Autodesk Inventor part; units mm, degrees
ref_plane "YZ Plane" through (0, 0, 0) normal (1, 0, 0) x (0, 1, 0)
ref_plane "XZ Plane" through (0, 0, 0) normal (0, 1, 0) x (-1, 0, 0)
ref_plane "XY Plane" through (0, 0, 0) normal (0, 0, 1) x (1, 0, 0)
sketch "Sketch1" plane through (0, 0, 0) normal (0, 1, 0) x (-1, 0, 0)
  line L0 (101.6, 38.1) -> (-101.6, 38.1) construction
  line L1 (-101.6, 38.1) -> (-101.6, -38.1) construction
  line L2 (-101.6, -38.1) -> (101.6, -38.1) construction
  line L3 (101.6, -38.1) -> (101.6, 38.1) construction
  line L4 (101.6, 38.1) -> (-101.6, -38.1) construction
  line L5 (-101.6, 38.1) -> (101.6, -38.1) construction
  line L6 (-28.575, 66.675) -> (28.575, 66.675) construction
  line L7 (28.575, 66.675) -> (28.575, 9.525)
  line L8 (28.575, 9.525) -> (-28.575, 9.525) construction
  line L9 (-28.575, 9.525) -> (-28.575, 66.675)
  line L10 (-28.575, 66.675) -> (28.575, 9.525) construction
  line L11 (28.575, 66.675) -> (-28.575, 9.525) construction
  circle A0 centre (-38.1, 50.8) radius 3.175
  line L12 (0, 38.1) -> (0, -38.1) construction
  circle A1 centre (-38.1, 50.8) radius 9.525
  line L13 (-38.1, 60.325) -> (-28.575, 60.325)
  circle A2 centre (38.1, 50.8) radius 3.175
  circle A3 centre (38.1, 50.8) radius 9.525
  line L14 (38.1, 60.325) -> (28.575, 60.325)
  circle A4 centre (-76.2, -38.1) radius 1.7526
  circle A5 centre (-95.25, 3.175) radius 1.7526
  circle A6 centre (76.2, -38.1) radius 1.7526
  circle A7 centre (95.25, 3.175) radius 1.7526
  line L15 (-101.6, -38.1) -> (-101.6, 6.35)
  line L16 (-101.6, 6.35) -> (-44.4797, 57.8728)
  line L17 (101.6, -38.1) -> (101.6, 6.35)
  line L18 (101.6, 6.35) -> (44.4797, 57.8728)
  line L19 (-42.6417, 42.4275) -> (-87.975, 1.5367) construction
  line L20 (-87.975, 1.5367) -> (-87.975, -38.1)
  line L21 (87.975, -38.1) -> (87.975, 1.5367)
  line L22 (87.975, 1.5367) -> (42.6417, 42.4275) construction
  line L23 (0, -38.1) -> (-95.25, -38.1) construction
  line L24 (0, -38.1) -> (95.25, -38.1) construction
  circle A8 centre (-60.325, 35.0287) radius 1.7526
  circle A9 centre (-33.3375, 31.75) radius 1.7526
  line L25 (-38.1, 0) -> (-38.1, 41.275)
  line L26 (-38.1, 0) -> (0, 0) construction
  circle A10 centre (60.325, 35.0287) radius 1.7526
  circle A11 centre (33.3375, 31.75) radius 1.7526
  line L27 (38.1, 0) -> (38.1, 41.275)
  line L28 (38.1, 0) -> (0, 0) construction
  line L29 (-87.975, 0) -> (-65.115, 0)
  line L30 (-65.115, 0) -> (-65.115, -31.75)
  line L31 (-65.115, -31.75) -> (-87.975, -31.75)
  line L32 (-101.6, -38.1) -> (101.6, -38.1) construction
  line L33 (101.6, -38.1) -> (101.6, 19.05)
  line L34 (101.6, 19.05) -> (-101.6, 19.05) construction
  line L35 (-101.6, 19.05) -> (-101.6, -38.1)
  line L36 (-101.6, 19.05) -> (-87.5203, 19.05) construction
  line L37 (87.5203, 19.05) -> (101.6, 19.05) construction
  circle A12 centre (-38.1, 0) radius 3.175 construction
  circle A13 centre (-38.1, 0) radius 6.35 construction
  circle A14 centre (38.1, 0) radius 3.175 construction
  circle A15 centre (38.1, 0) radius 6.35 construction
  circle A16 centre (28.575, 9.525) radius 1.7526
  circle A17 centre (28.575, 9.525) radius 4.7625
  arc A18 (17.0773, 9.525) -> (28.575, 21.0227) centre (17.0773, 21.0227) ccw
  circle A19 centre (-28.575, 9.525) radius 1.7526
  circle A20 centre (-28.575, 9.525) radius 4.7625
  arc A21 (-28.575, 21.0227) -> (-17.0773, 9.525) centre (-17.0773, 21.0227) ccw
  arc A22 (31.4325, 5.715) -> (38.1, 19.05) centre (21.4312, 19.05) ccw
  arc A23 (-38.1, 19.05) -> (-31.4325, 5.715) centre (-21.4312, 19.05) ccw
  line L38 (-61.94, -38.1) -> (-61.94, 25.0204)
  line L39 (87.975, 0) -> (65.115, 0)
  line L40 (65.115, 0) -> (65.115, -31.75)
  line L41 (65.115, -31.75) -> (87.975, -31.75)
  line L42 (61.94, -38.1) -> (61.94, 25.0204)
  line L43 (-28.575, 4.7625) -> (28.575, 4.7625)
  line L44 (101.6, -31.75) -> (-101.6, -31.75)
  line L45 (-101.6, -31.75) -> (-101.6, -44.45) construction
  line L46 (-101.6, -44.45) -> (101.6, -44.45)
  line L47 (101.6, -44.45) -> (101.6, -31.75) construction
  circle A24 centre (0, -38.1) radius 1.7526
  circle A25 centre (38.1, -38.1) radius 1.7526
  circle A26 centre (-38.1, -38.1) radius 1.7526
  line L48 (101.6, -38.1) -> (76.2, -44.45)
  line L49 (-101.6, -38.1) -> (-76.2, -44.45)
  line L50 (76.2, -38.1) -> (76.2, -44.45) construction
  line L51 (-76.2, -38.1) -> (-76.2, -44.45) construction
  line L52 (59.1924, 41.2769) -> (32.488, 36.4361)
  circle A27 centre (60.325, 35.0287) radius 6.35
  circle A28 centre (33.3375, 31.75) radius 4.7625
  line L53 (-59.1924, 41.2769) -> (-32.488, 36.4361)
  circle A29 centre (-60.325, 35.0287) radius 6.35
  circle A30 centre (-33.3375, 31.75) radius 4.7625
  line L54 (-87.975, 0) -> (-65.115, 0)
  line L55 (-65.115, 0) -> (-65.115, -3.175)
  line L56 (-65.115, -3.175) -> (-87.975, -3.175)
  line L57 (-87.975, -3.175) -> (-87.975, 0)
  line L58 (-65.115, -15.875) -> (-87.975, -15.875) construction
  line L59 (-65.115, -28.575) -> (-87.975, -28.575)
  line L60 (-84.8, -38.1) -> (-84.8, 0.1248)
  line L61 (65.115, -3.175) -> (87.975, -3.175)
  line L62 (65.115, -15.875) -> (87.975, -15.875) construction
  line L63 (65.115, -28.575) -> (87.975, -28.575)
  line L64 (84.8, -38.1) -> (84.8, 0.1248)
  line L65 (-31.75, -31.75) -> (31.75, -31.75)
  line L66 (31.75, -31.75) -> (31.75, 0)
  line L67 (31.75, 0) -> (-31.75, 0)
  line L68 (-31.75, 0) -> (-31.75, -31.75)
  circle A31 centre (71.465, 12.7) radius 3.175
  circle A32 centre (-71.465, 12.7) radius 3.175
  line L69 (-17.0773, 9.525) -> (17.0773, 9.525)
  point P0 (28.575, 38.1)
  point P1 (-28.575, 38.1)
  point P2 (28.575, 60.325)
  point P3 (44.4797, 57.8728)
  point P4 (101.6, -15.875)
  point P5 (38.1, 41.275)
  point P6 (-87.975, -31.75)
  point P7 (-101.6, 6.35)
  point P8 (101.6, 6.35)
  point P9 (31.75, 0)
  point P10 (38.1, 6.35)
  point P11 (-38.1, 6.35)
  point P12 (-31.75, 0)
  point P13 (87.975, 0)
  point P14 (61.94, 25.0204)
  point P15 (-17.0773, 9.525)
  point P16 (-28.575, 21.0227)
  point P17 (-38.1, 19.05)
  point P18 (-31.4325, 5.715)
  point P19 (-21.8502, 0)
  point P20 (21.8502, 0)
  point P21 (-25.2074, 12.8926)
  point P22 (-28.575, 14.2875)
  point P23 (-23.8125, 9.525)
  point P24 (-28.575, 50.8)
  point P25 (25.2074, 12.8926)
  point P26 (28.575, 14.2875)
  point P27 (23.8125, 9.525)
  point P28 (28.575, 50.8)
  point P29 (26.8224, 9.525)
  point P30 (28.575, 11.2776)
  point P31 (61.94, -31.75)
  point P32 (-61.94, -31.75)
  point P33 (-28.575, 31.75)
  point P34 (-64.5781, 39.7439)
  point P35 (64.5781, 39.7439)
  point P36 (28.575, 31.75)
  point P37 (-84.8, -3.175)
  point P38 (-84.8, -28.575)
  point P39 (84.8, -3.175)
  point P40 (84.8, -28.575)
  point P41 (31.75, -31.75)
  point P42 (-101.6, -31.75)
  point P43 (31.75, -31.75)
  point P44 (-26.8224, 9.525)
  point P45 (-28.575, 11.2776)
  point P46 (-39.8526, -38.1)
  point P47 (-36.3474, -38.1)
  point P48 (-1.7526, -38.1)
  point P49 (1.7526, -38.1)
  point P50 (36.3474, -38.1)
  point P51 (39.8526, -38.1)
  dimension "d0" = 203.2
  dimension "d1" = 76.2
  dimension "d4" = 57.15
  dimension "d6" = 6.35
  dimension "d7" = 38.1
  dimension "d8" = 19.05
  dimension "d10" = 3.5052
  dimension "d11" = 3.5052
  dimension "d12" = 0
  dimension "d14" = 25.4
  dimension "d15" = 6.35
  dimension "d20" = 50.8
  dimension "d21" = 41.275
  dimension "d22" = 44.45
  dimension "d24" = 12.7
  dimension "d25" = 13.625
  dimension "d26" = 12.7
  dimension "d27" = 13.625
  dimension "d31" = 3.5052
  dimension "d32" = 3.5052
  dimension "d33" = 6.35
  dimension "d34" = 31.75
  dimension "d35" = 4.7625
  dimension "d36" = 22.225
  dimension "d37" = 9.525
  dimension "d39" = 31.75
  dimension "d40" = 6.35
  dimension "d42" = 57.15
  dimension "d43" = 6.35
  dimension "d44" = 9.525
  dimension "d45" = 9.525
  dimension "d46" = 12.7
  dimension "d104" = 3.5052
  dimension "d105" = 9.525
  dimension "d106" = 3.175
  dimension "d107" = 22.86
  dimension "d123" = 88.9
  dimension "d124" = 12.7
  dimension "d125" = 3.5052
  dimension "d126" = 3.5052
  dimension "d127" = 38.1
  dimension "d128" = 28.575
  dimension "d129" = 3.175
  dimension "d130" = 3.175
  dimension "d131" = 31.75
  dimension "d132" = 31.75
  dimension "d133" = 31.75
  dimension "d135" = 6.35
  dimension "d136" = 12.7
  dimension "d137" = 9.525
extrude "Extrusion1" add sketch "Sketch1" along normal blind 3.175 contours A28 L27 A22 A17 L7 | A28 | L7 A17 A18 | L52 L27 A28 | L27 L52 A27 L18 L17 L44 L21 L39 L40 L66 L67 L68 L30 L29 L20 L15 L16 A29 L53 L25 A23 A20 L43 A17 A22 | A27 | A17 | A17 L43 A20 A21 L69 A18 | L17 L48 L46 L49 L15 L44 L31 L41 | A20 | L41 L64 L63 L21 | A23 L25 A30 L9 A20 | A20 L9 A21 | L63 L64 L61 L21 | L41 L40 L63 L64 | L61 L64 L39 L21 | L63 L40 L61 L64 | L25 L53 A30 | A30 | L61 L40 L39 L64 | A29 | L20 L59 L60 L31 | L20 L56 L60 L59 | L60 L59 L30 L31 | L20 L29 L60 L56 | L60 L56 L30 L59 | L60 L29 L30 L56
fillet "Fillet1" radius 6.35 6 edges at (101.6, 1.5875, -38.1) (101.6, 1.5875, 6.35) (-101.6, 1.5875, 6.35) (76.2, 1.5875, -44.45) (-76.2, 1.5875, -44.45) (-101.6, 1.5875, -38.1)
fillet "Fillet5" radius 6.35 4 edges at (31.75, 1.5875, 0) (-31.75, 1.5875, 0) (-31.75, 1.5875, -31.75) (31.75, 1.5875, -31.75)
equation "\"d35\" = 0.5 * d37"
properties part number "Chassis" material "UHMW, White"
CAD build for the part. Positions are in the model's coordinates, mm. A direction names the side the tool comes from. Round coordinates to 2 decimals unless told otherwise and drop trailing zeros. Write each loop counter-clockwise with the first axis right and the second up, starting at its lowest first coordinate (ties: lowest second). Pieces come first, ordered by that corner, then holes. Notation, with made-up numbers: M 85.5,-21 L 108.5,-21 A32 cw 108.5,15 Z; hole C 35.25,89 d11. An arc over 180 degrees is marked long. One line per question, with ' | ' between items.
1. Cut at B-B on x = -10.5. Write the cut outline in (y, z) (3 decimals), and give its area (3 significant figures).
Working result:
outline: M 0,-44.45 L 3.175,-44.45 L 3.175,-31.75 L 0,-31.75 Z; M 0,0 L 3.175,0 L 3.175,9.525 L 0,9.525 Z | area: 70.6 mm2
2. Cut at A-A on z = -20.5. Write the cut outline in (x, y) (3 decimals).
Working result:
outline: M -101.6,0 L -31.75,0 L -31.75,3.175 L -101.6,3.175 Z; M 31.75,0 L 101.6,0 L 101.6,3.175 L 31.75,3.175 Z
3. Pin check, flat tip, straight feed: pin 1 Ø5 at (x, z) = (-65, 20.5) entering from -Y. Stop position of the tip, or through.
Working result:
pin 1: y = 0
4. Which spindle directions (+Z, -Z, +X, -X, +Y, -Y) get a long thin tool onto all of the face, cutting with end or side? Do faces 4 (the cylindrical face through (100.291, 1.61, -37.003)), 5 (the cylindrical face through (29.84, 1.61, -1.81)), 6 (the cylindrical face through (-25.296, 1.565, 12.982)). Say none if no direction does.
Working result:
face 4: -Z, +X, +Y, -Y | face 5: +Y, -Y | face 6: +Z, +Y, -Y
5. Cut at C-C on y = 2.35. Count the separate pieces of the cut face and the enclosed holes in it, and give its area (3 significant figures).
Working result:
separate pieces: 1 | enclosed holes: 16 | area: 11,800 mm2
6. Cut at D-D on x = -47. Write the cut outline in (y, z) (3 decimals).
Working result:
outline: M 0,-44.45 L 3.175,-44.45 L 3.175,39.067 L 0,39.067 Z
7. Probe L1, parallel to Z at x = 0, y = 0.85 (3 decimals); L2, parallel to Z at x = -4.5, y = 0.55 (3 decimals); L3, parallel to X at y = 2.4, z = -39. List the from-to ranges inside material, lowest first. Write a range as from..to.
Working result:
L1: -44.45..-39.853, -36.347..-31.75, 0..9.525 | L2: -44.45..-31.75, 0..9.525 | L3: -97.7..-77.7, -74.7..-39.6, -36.6..-1.5, 1.5..36.6, 39.6..74.7, 77.7..97.7
8. Mould opens along X. For faces 1 (the cylindrical face through (58.706, 1.565, 35.7)), 2 (the flat face through (87.013, 1.565, -41.747)), 3 (the flat face through (-82.29, 1.57, 23.77)) say: pulls with the +X half, pulls with the -X half, needs draft (parallel to the pull), parting line crosses it, or undercut.
Working result:
face 1: undercut | face 2: pulls with the +X half | face 3: pulls with the -X half
